Geometry: final body of the model. Coordinates: model frame, mm. A direction names the side the tool comes from. Give positions to 0.01 mm unless a question says otherwise; leave off trailing zeros. Write each loop counter-clockwise with the first axis right and the second up, starting at its lowest first coordinate (ties: lowest second). Pieces come first, ordered by that corner, then holes. Notation, with made-up numbers: M 72,-34.75 L 128,-34.75 A14 ccw 128,-20.75 Z; hole C 50,-12.5 d2. An arc over 180 degrees is marked long. Use a Markdown table: item, result. Add a question column.
1) Line query: line 1 (Z direction, x = 47, y = 55); line 2 (X direction, y = 53, z = 70); line 3 (Z direction, x = 45.5, y = 35). Output: solid intervals per line, ascending.
2) Set-up query: faces 5 (the cylindrical face through (12.33, -72.98, 52.69)), 6 (the flat face through (44.45, -10, 19)). Return all of +Z, -Z, +X, -X, +Y, -Y with unobstructed straight access to the full face (end or side cutting, diameter ignored); none if empty.
3) Pin query (flat end, axial travel): pin 1 (6.5 mm diameter, centred on x = -14.1, z = 44.41, fed in from +Y); pin 2 (4.5 mm diameter, centred on y = 18.83, z = 110.41, fed in from -X); pin 3 (1.5 mm diameter, centred on y = -60.5, z = 23, fed in from -X). Return the tip coordinate at first contact, or that it passes through.
4) Section D-D on y = 10.5. Return the cut outline in (x, z), then the cut area to 3 significant figures.
5) Section B-B on y = -22. Return the cut outline in (x, z).
6) Section A-A on z = 51. Return the cut outline in (x, y).
7) Section C-C on z = 99.5. Return the cut outline in (x, y), then the cut area to 3 significant figures.
8) Draft query along X for faces 1 (the cylindrical face through (-13.558, -72.981, 73.148)), 2 (the cylindrical face through (-4.56, -72.98, 41.66)), 3 (the flat face through (10.363, -72.981, 102.498)), 4 (the flat face through (8, -69.85, 59)). Return one class per face: +X half, -X half, draft (parallel to the pull), parting line (faces both ways), or undercut.
```python
from build123d import *

# Parameters (mm, degrees)
BOSS_EXTRUDE1_DEPTH = 120
CUT_EXTRUDE1_DEPTH  = 6.35
SKETCH4_R           = 2.5
CUT_EXTRUDE2_DEPTH  = 6.35
SKETCH5_R           = 2
SKETCH5_R_2         = 42.5
CUT_EXTRUDE4_DEPTH  = 6.35
CUT_EXTRUDE8_DEPTH  = 6.35


with BuildPart() as part:
    # Sketch2 → Boss-Extrude1 (new body)
    with BuildSketch(Plane.XY):
        with BuildLine():
            Line((-50.8, -76.2), (50.8, -76.2))
            Line((50.8, -76.2), (50.8, 76.2))
            Line((50.8, 76.2), (47.625, 76.2))
            ThreePointArc((47.625, 76.2), (45.37993597, 75.27006403), (44.45, 73.025))
            Line((44.45, 73.025), (44.45, -57.15))
            ThreePointArc((44.45, -57.15), (40.730256121, -66.130256121), (31.75, -69.85))
            Line((31.75, -69.85), (-47.625, -69.85))
            ThreePointArc((-47.625, -69.85), (-49.87006403, -70.77993597), (-50.8, -73.025))
            Line((-50.8, -73.025), (-50.8, -76.2))
        make_face()
    extrude(amount=BOSS_EXTRUDE1_DEPTH)

    # Sketch3 → Cut-Extrude1 (cut)
    with BuildSketch(Plane(origin=(0, -69.85, 0), x_dir=(1, 0, 0), z_dir=(0, 1, 0))):
        with BuildLine():
            Line((-5.1, -35.5), (25.4, 0))
            Line((25.4, 0), (-50.8, 0))
            Line((-50.8, 0), (-50.8, -120))
            Line((-50.8, -120), (25.4, -120))
            Line((25.4, -120), (-5.1, -84.5))
            ThreePointArc((-5.1, -84.5), (-29.6, -60), (-5.1, -35.5))
        make_face()
    extrude(amount=-CUT_EXTRUDE1_DEPTH, mode=Mode.SUBTRACT)

    # Sketch4 → Cut-Extrude2 (cut)
    with BuildSketch(Plane(origin=(0, -69.85, 0), x_dir=(1, 0, 0), z_dir=(0, 1, 0))):
        with Locations(Location((-5.1, -44.1, 0), (0, 0, 180))):
            Circle(SKETCH4_R)
        with Locations(Location((8.66980392, -67.95, 0), (0, 0, 180))):
            Circle(SKETCH4_R)
        with Locations(Location((-18.86980392, -67.95, 0), (0, 0, 180))):
            Circle(SKETCH4_R)
        with Locations(Location((3.9, -44.411542732, 0), (0, 0, 180))):
            Circle(SKETCH4_R)
        with Locations(Location((10.488457268, -51, 0), (0, 0, 180))):
            Circle(SKETCH4_R)
        with Locations(Location((12.9, -60, 0), (0, 0, 180))):
            Circle(SKETCH4_R)
        with Locations(Location((3.9, -75.588457268, 0), (0, 0, 180))):
            Circle(SKETCH4_R)
        with Locations(Location((-5.1, -78, 0), (0, 0, 180))):
            Circle(SKETCH4_R)
        with Locations(Location((-14.1, -75.588457268, 0), (0, 0, 180))):
            Circle(SKETCH4_R)
        with Locations(Location((-23.1, -60, 0), (0, 0, 180))):
            Circle(SKETCH4_R)
        with Locations(Location((-20.688457268, -51, 0), (0, 0, 180))):
            Circle(SKETCH4_R)
        with Locations(Location((-14.1, -44.411542732, 0), (0, 0, 180))):
            Circle(SKETCH4_R)
    extrude(amount=-CUT_EXTRUDE2_DEPTH, mode=Mode.SUBTRACT)

    # Sketch5 → Cut-Extrude4 (cut)
    with BuildSketch(Plane.ZY.offset(-44.45)):
        with Locations(Location((60, 55.45, 0), (0, 0, 270))):
            Circle(SKETCH5_R)
        with Locations(Location((91.152618372, 45.327900702, 0), (0, 0, 270))):
            Circle(SKETCH5_R)
        with Locations(Location((110.405995364, 18.827900702, 0), (0, 0, 270))):
            Circle(SKETCH5_R)
        with Locations(Location((110.405995364, -13.927900702, 0), (0, 0, 270))):
            Circle(SKETCH5_R)
        with Locations(Location((91.152618372, -40.427900702, 0), (0, 0, 270))):
            Circle(SKETCH5_R)
        with Locations(Location((60, -50.55, 0), (0, 0, 270))):
            Circle(SKETCH5_R)
        with Locations(Location((28.847381629, -40.427900702, 0), (0, 0, 270))):
            Circle(SKETCH5_R)
        with Locations(Location((9.594004636, -13.927900702, 0), (0, 0, 270))):
            Circle(SKETCH5_R)
        with Locations(Location((9.594004636, 18.827900702, 0), (0, 0, 270))):
            Circle(SKETCH5_R)
        with Locations(Location((28.847381629, 45.327900702, 0), (0, 0, 270))):
            Circle(SKETCH5_R)
        with Locations(Location((60, 2.45, 0), (0, 0, 270))):
            Circle(SKETCH5_R_2)
    extrude(amount=-CUT_EXTRUDE4_DEPTH, mode=Mode.SUBTRACT)

    # Sketch6 → Cut-Extrude8 (cut)
    with BuildSketch(Plane.ZY.offset(-44.45)):
        with BuildLine():
            Line((0, 76.2), (0, 2.45))
            ThreePointArc((0, 2.45), (60, 62.45), (120, 2.45))
            Line((120, 2.45), (120, 76.2))
            Line((120, 76.2), (0, 76.2))
        make_face()
    extrude(amount=-CUT_EXTRUDE8_DEPTH, mode=Mode.SUBTRACT)


solid = part.part
```
Found:
| question | item | result |
|---|---|---|
| 1 | line 1 | 31.04 to 58.05, 61.95 to 88.96 |
| 1 | line 2 | 44.45 to 50.8 |
| 1 | line 3 | 9.6 to 32.67, 87.33 to 110.4 |
| 2 | face 5 | +Y, -Y |
| 2 | face 6 | +Z, -Z, -X, +Y |
| 3 | pin 1 | y = -69.85 |
| 3 | pin 2 | x = 44.45 |
| 3 | pin 3 | x = 43.77 |
| 4 | outline | M 44.45,0.54 L 50.8,0.54 L 50.8,18.27 L 44.45,18.27 Z; M 44.45,101.73 L 50.8,101.73 L 50.8,119.46 L 44.45,119.46 Z |
| 4 | area | 225 mm² |
| 5 | outline | M 44.45,0 L 50.8,0 L 50.8,25.24 L 44.45,25.24 Z; M 44.45,94.76 L 50.8,94.76 L 50.8,120 L 44.45,120 Z |
| 6 | outline | M -27.89,-76.2 L -23.19,-76.2 L -23.19,-69.85 L -27.89,-69.85 Z; M -18.19,-76.2 L 7.99,-76.2 L 7.99,-69.85 L -18.19,-69.85 Z; M 12.99,-76.2 L 50.8,-76.2 L 50.8,-39.09 L 44.45,-39.09 L 44.45,-57.15 A12.7 cw 31.75,-69.85 L 12.99,-69.85 Z; M 44.45,43.99 L 50.8,43.99 L 50.8,61.77 L 44.45,61.77 Z |
| 7 | outline | M 7.79,-76.2 L 50.8,-76.2 L 50.8,-13.23 L 44.45,-13.23 L 44.45,-57.15 A12.7 cw 31.75,-69.85 L 7.79,-69.85 Z; M 44.45,18.13 L 50.8,18.13 L 50.8,47.61 L 44.45,47.61 Z |
| 7 | area | 854 mm² |
| 8 | face 1 | undercut |
| 8 | face 2 | undercut |
| 8 | face 3 | -X half |
| 8 | face 4 | draft |
